Check sheet for the drawn part. Datum: minimum x, y, z corner. Units: mm. A direction names the side the tool comes from. Coordinates: 2 decimals unless noted, no trailing zeros. Order: outer loops, then holes, each group sorted by start corner. A loop starts at its lowest first (then second) coordinate and runs counter-clockwise, first axis right, second up. Notation, with made-up numbers: (37.5, 52) - (65.5, 52) arc R25 cw to (65.5, 79) - close; hole circle Ø3 at (-24, 73.5). An arc over 180 degrees is marked (long way). Return JSON: item names as keys, results as strings. Group by question number.
Item 1: Tool access check on the marked faces 1, 2 and 3. Record the directions out of +Z, -Z, +X, -X, +Y, -Y that give a thin tool (end or side, any length) a straight path to the whole face; none if there is none.
Item 2: Section check A-A on x = 37.5. Enter the section's corners in (y, z), then the cut area to 3 significant figures.
Item 3: Section check C-C on y = 61. Enter the section's corners in (x, z), then the cut area to 3 significant figures.
Item 4: Scan lines: probe 1 along X at (y, z) = (26, 30); probe 2 along Z at (x, y) = (37, 54); probe 3 along Z at (x, y) = (44.5, 68). Record each from-to range of solid material in increasing order.
Item 5: Draft check along Z on the marked faces 4, 5 and 6. Enter one of: pulls with the +Z half, pulls with the -Z half, needs draft (parallel to the pull), parting line crosses it, or undercut.
Item 6: Section check D-D on z = 6.5. Enter the section's corners in (x, y), then the cut area to 3 significant figures.
Item 7: Section check B-B on z = 27. Enter the section's corners in (x, y), then the cut area to 3 significant figures.
Item 8: Gauge pin test, flat ends, axial feed: pin 1 (1.5 mm diameter, centred on x = 62.5, y = 65.5, fed in from +Z); pin 2 (4 mm diameter, centred on y = 58.5, z = 28.5, fed in from -X); pin 3 (6 mm diameter, centred on x = 23, y = 47.5, fed in from +Z); pin 4 (2 mm diameter, centred on x = 66.5, z = 38.5, fed in from -Y). Record the tip position at first contact, or that the pin passes through.
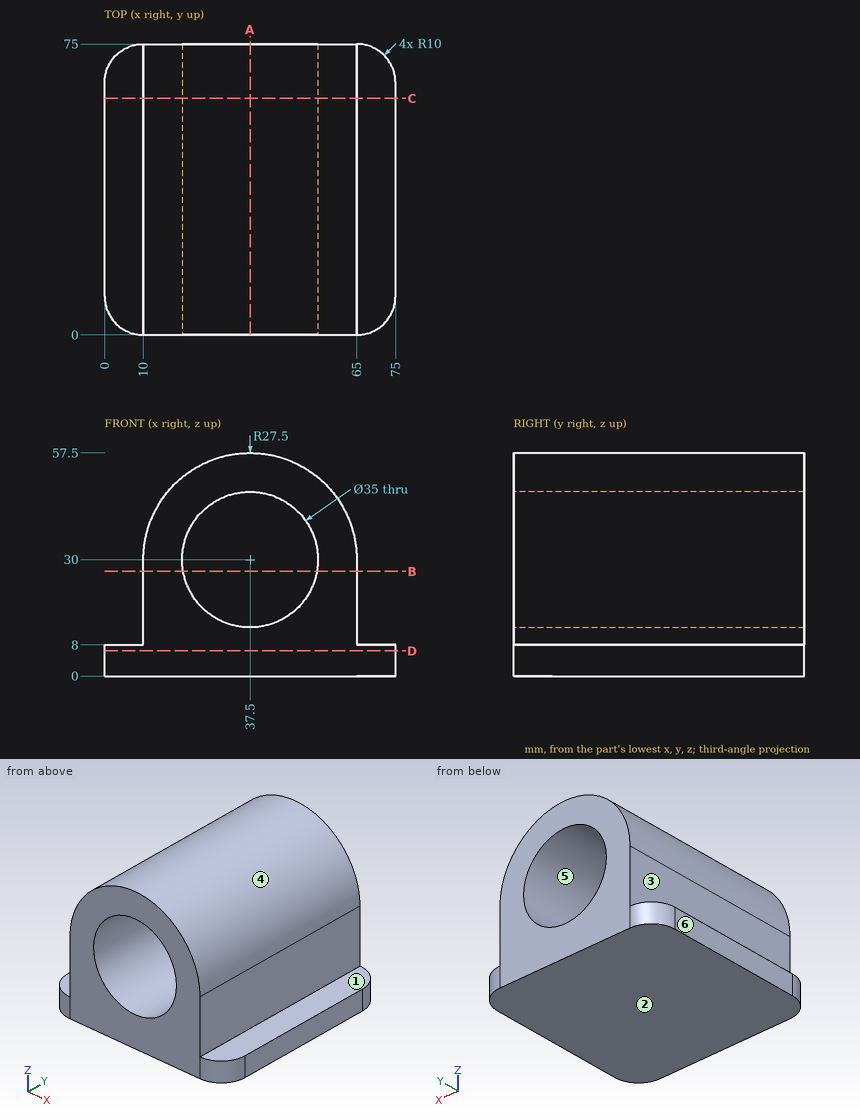
Computed:
{
 "1": {"face 1": "+Z, +X, +Y, -Y", "face 2": "-Z, +X, -X, +Y, -Y", "face 3": "+Z, -X, +Y, -Y"},
 "2": {"outline": "(0, 0) - (75, 0) - (75, 12.5) - (0, 12.5) - close; (0, 47.5) - (75, 47.5) - (75, 57.5) - (0, 57.5) - close", "area": "1,690 mm²"},
 "3": {"outline": "(0, 0) - (75, 0) - (75, 8) - (65, 8) - (65, 30) arc R27.5 ccw to (10, 30) - (10, 8) - (0, 8) - close; hole circle Ø35 at (37.5, 30)", "area": "2,040 mm²"},
 "4": {"probe 1": "x = 10 to 20, 55 to 65", "probe 2": "z = 0 to 12.51, 47.49 to 57.5", "probe 3": "z = 0 to 13.96, 46.04 to 56.59"},
 "5": {"face 4": "pulls with the +Z half", "face 5": "undercut", "face 6": "needs draft"},
 "6": {"outline": "(0, 10) arc R10 ccw to (10, 0) - (65, 0) arc R10 ccw to (75, 10) - (75, 65) arc R10 ccw to (65, 75) - (10, 75) arc R10 ccw to (0, 65) - close", "area": "5,540 mm²"},
 "7": {"outline": "(10, 0) - (20.26, 0) - (20.26, 75) - (10, 75) - close; (54.74, 0) - (65, 0) - (65, 75) - (54.74, 75) - close", "area": "1,540 mm²"},
 "8": {"pin 1": "stops at z = 42.97", "pin 2": "stops at x = 10", "pin 3": "stops at z = 54.98", "pin 4": "passes through"}
}
